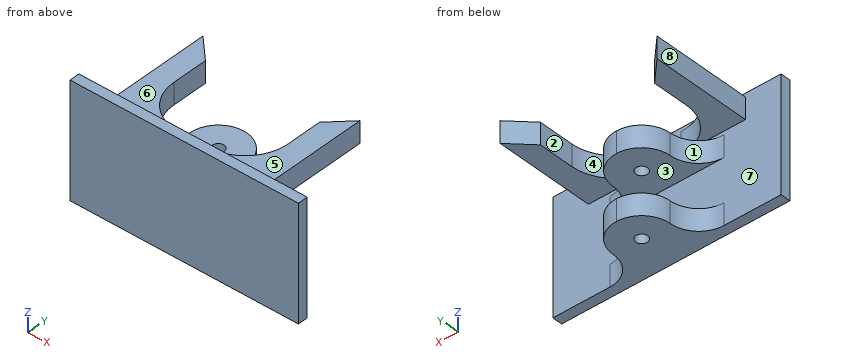
from build123d import *

# Parameters (mm, degrees)
SKETCH1_W           = 160
SKETCH1_H           = 60
BOSS_EXTRUDE1_DEPTH = 7
SKETCH2_W           = 40
SKETCH2_H           = 60
BOSS_EXTRUDE2_DEPTH = 40
FILLET1_R           = 20
SKETCH3_W           = 30
SKETCH3_H           = 40
CUT_EXTRUDE1_DEPTH  = 40
SKETCH4_R           = 4.15
CUT_EXTRUDE2_DEPTH  = 178.225844616
FILLET2_R           = 20
SKETCH5_W           = 160
SKETCH5_H           = 7
BOSS_EXTRUDE3_DEPTH = 20
SKETCH6_W           = 15
SKETCH6_H           = 15
BOSS_EXTRUDE4_DEPTH = 70
FILLET3_R           = 30
CHAMFER1_SIZE       = 15


with BuildPart() as part:
    # Sketch1 → Boss-Extrude1 (new body)
    with BuildSketch(Plane(origin=(0, 0, 0), x_dir=(1, 0, 0), z_dir=(0, 1, 0))):
        with Locations((-80, 30)):
            Rectangle(SKETCH1_W, SKETCH1_H)
    extrude(amount=BOSS_EXTRUDE1_DEPTH)

    # Sketch2 → Boss-Extrude2 (add)
    with BuildSketch(Plane(origin=(0, 7, 0), x_dir=(1, 0, 0), z_dir=(0, 1, 0))):
        with Locations((-80, 30)):
            Rectangle(SKETCH2_W, SKETCH2_H)
    extrude(amount=BOSS_EXTRUDE2_DEPTH)

    # Fillet1
    fillet1_edges = [part.edges().sort_by_distance(p)[0] for p in [
        (-60, 47, -30),
        (-100, 47, -30),
    ]]
    fillet(fillet1_edges, radius=FILLET1_R - 0.0001)  # a hair under: the kernel refuses the full size

    # Sketch3 → Cut-Extrude1 (cut)
    with BuildSketch(Plane(origin=(-60, 0, 0), x_dir=(0, 0, -1), z_dir=(1, 0, 0))):
        with Locations((30, 27)):
            Rectangle(SKETCH3_W, SKETCH3_H)
    extrude(amount=-CUT_EXTRUDE1_DEPTH, mode=Mode.SUBTRACT)

    # Sketch4 → Cut-Extrude2 (cut, through all)
    with BuildSketch(Plane.XY):
        with Locations((-80, 27)):
            Circle(SKETCH4_R)
    extrude(amount=-CUT_EXTRUDE2_DEPTH, mode=Mode.SUBTRACT)

    # Fillet2
    fillet2_edges = [part.edges().sort_by_distance(p)[0] for p in [
        (-100, 7, -7.5),
        (-100, 7, -52.5),
        (-60, 7, -7.5),
        (-60, 7, -52.5),
    ]]
    fillet(fillet2_edges, radius=FILLET2_R)

    # Sketch5 → Boss-Extrude3 (add)
    with BuildSketch(Plane.XY):
        with Locations((-80, 3.5)):
            Rectangle(SKETCH5_W, SKETCH5_H)
    extrude(amount=BOSS_EXTRUDE3_DEPTH)

    # Sketch6 → Boss-Extrude4 (add)
    with BuildSketch(Plane(origin=(0, 7, 0), x_dir=(1, 0, 0), z_dir=(0, 1, 0))):
        with Locations((-127.5, -10)):
            Rectangle(SKETCH6_W, SKETCH6_H)
        with Locations((-32.5, -10)):
            Rectangle(SKETCH6_W, SKETCH6_H)
    extrude(amount=BOSS_EXTRUDE4_DEPTH)

    # Fillet3
    fillet3_edges = [part.edges().sort_by_distance(p)[0] for p in [
        (-120, 7, 10),
        (-40, 7, 10),
    ]]
    fillet(fillet3_edges, radius=FILLET3_R)

    # Chamfer1
    chamfer1_edges = [part.edges().sort_by_distance(p)[0] for p in [
        (-40, 77, 10),
        (-120, 77, 10),
    ]]
    chamfer(chamfer1_edges, length=CHAMFER1_SIZE - 0.0001)  # a hair under: the kernel refuses the full size


solid = part.part
Geometry check sheet. Reference: the model listing, model coordinates, mm. Face numbers are marked on the shaded views. A direction names the side the tool comes from. Give positions to 0.01 mm unless a question says otherwise; leave off trailing zeros. Loops run counter-clockwise (first coordinate to the right, second up) from the corner with the lowest first, then second, coordinate; pieces in that order, holes last.
(1) Thickness scan on L1, parallel to Z at x = -103.5, y = 8; L2, parallel to Y at x = -80, z = -10; L3, parallel to Z at x = -86, y = 10. Record the ranges inside material, lowest first.
From the geometry:
L1: z = -60 to -45, -15 to 0, 2.5 to 17.5
L2: y = 0 to 22.85, 31.15 to 47
L3: z = -60 to -45, -15 to 0
(2) Section check B-B on y = 20. Record the cut outline in (x, z) (3 decimals).
From the geometry:
outline: (-135, 2.5) - (-114.718, 2.5) - (-114.718, 17.5) - (-135, 17.5) - close; (-101.265, -60) - (-58.735, -60) - (-58.735, -45) - (-101.265, -45) - close; (-101.265, -15) - (-58.735, -15) - (-58.735, 0) - (-101.265, 0) - close; (-45.282, 2.5) - (-25, 2.5) - (-25, 17.5) - (-45.282, 17.5) - close
(3) Release check for a two-part mould opening along Z. For the marked faces 6, 7 and 8 record: released by +Z, released by -Z, zero draft, split by the parting line, or undercut.
From the geometry:
face 6: released by +Z
face 7: undercut
face 8: zero draft
(4) Depth check by flat-ended pin: pin 1 Ø10 at (y, z) = (47, 3) entering from +X; pin 2 Ø2 at (y, z) = (21.5, -49.5) entering from +X; pin 3 Ø12 at (y, z) = (41.5, -15) entering from -X. Enter the tip coordinate at first touch or a pass-through.
From the geometry:
pin 1: stops at x = -25
pin 2: stops at x = -58.91
pin 3: stops at x = -98.1
(5) Section check D-D on x = -29.5. Record the cut outline in (y, z), then the cut area to 3 significant figures.
From the geometry:
outline: (0, -60) - (7, -60) - (7, 2.5) - (72.5, 2.5) - (72.5, 17.5) - (7, 17.5) - (7, 20) - (0, 20) - close
area: 1,540 mm2
(6) Set-up check for the marked faces 1, 2, 3, 4 and 5: record each of +Z, -Z, +X, -X, +Y, -Y from which the full face is reachable in a straight line by a thin tool's end or side.
From the geometry:
face 1: -Z, -X, +Y
face 2: +Z, -Z, +Y
face 3: +X, -X, +Y
face 4: +Z, +Y
face 5: +Z, +X, -X, +Y
